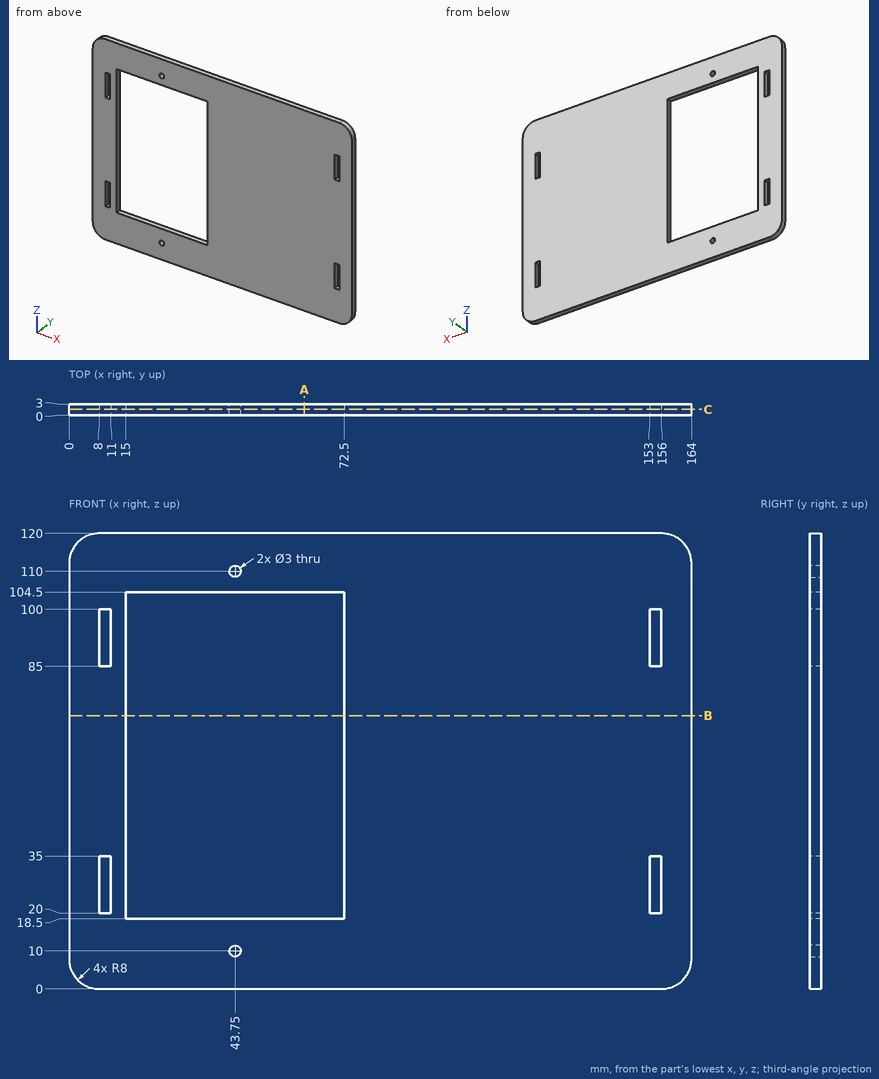
Study the drawing (mm; zero at the part's minimum x, y, z) and answer. Coordinates: 2 decimals unless noted, no trailing zeros. Write each loop counter-clockwise with the first axis right and the second up, starting at its lowest first coordinate (ties: lowest second). Pieces come first, ordered by that corner, then holes. Notation, with made-up numbers: (79, -27.5) - (113, -27.5) arc R17 cw to (113, -1.5) - close; hole circle Ø5 at (70.5, 78.25). An arc over 180 degrees is marked (long way). Return JSON: item names as keys, results as strings. Group by question number.
1. A cutting plane is placed at C-C, the plane y = 1.6. Give the number of separate pieces and of enclosed holes in the cut face, plus the area to 3 significant figures.
2. A cutting plane is placed at A-A, the plane x = 62. Determine the outline of the cut face in (y, z).
3. A cutting plane is placed at B-B, the plane z = 72. Determine the outline of the cut face in (x, y), plus the area to 4 significant figures.
4. Straight lines are drawn through the part: L1, parallel to Z at x = 155, y = 1.9; L2, parallel to Z at x = 43.75, y = 1.95; L3, parallel to X at y = 1.55, z = 10. For each, find the intervals that lie inside material, in ascending order.
Ans:
{
 "1": {"separate pieces": "1", "enclosed holes": "7", "area": "14,500 mm²"},
 "2": {"outline": "(0, 0) - (3, 0) - (3, 18.5) - (0, 18.5) - close; (0, 104.5) - (3, 104.5) - (3, 120) - (0, 120) - close"},
 "3": {"outline": "(0, 0) - (15, 0) - (15, 3) - (0, 3) - close; (72.5, 0) - (164, 0) - (164, 3) - (72.5, 3) - close", "area": "319.5 mm²"},
 "4": {"L1": "0 to 20, 35 to 85, 100 to 120", "L2": "0 to 8.5, 11.5 to 18.5, 104.5 to 108.5, 111.5 to 120", "L3": "0 to 42.25, 45.25 to 164"}
}
